Can you work these out from the drawing? Everything is in mm from the part's minimum corner. A direction names the side the tool comes from. Round coordinates to 2 decimals unless told otherwise and drop trailing zeros. Order: outer loops, then holes, each group sorted by start corner. A loop starts at its lowest first (then second) coordinate and runs counter-clockwise, first axis right, second up. Notation, with made-up numbers: (49.25, 75.5) -> (64.25, 75.5) arc R18 cw to (64.25, 92.5) -> close; hole circle Ø2 at (31, 22). An arc over 180 degrees is marked (long way). Use a Markdown table: item, result. Add a question column.
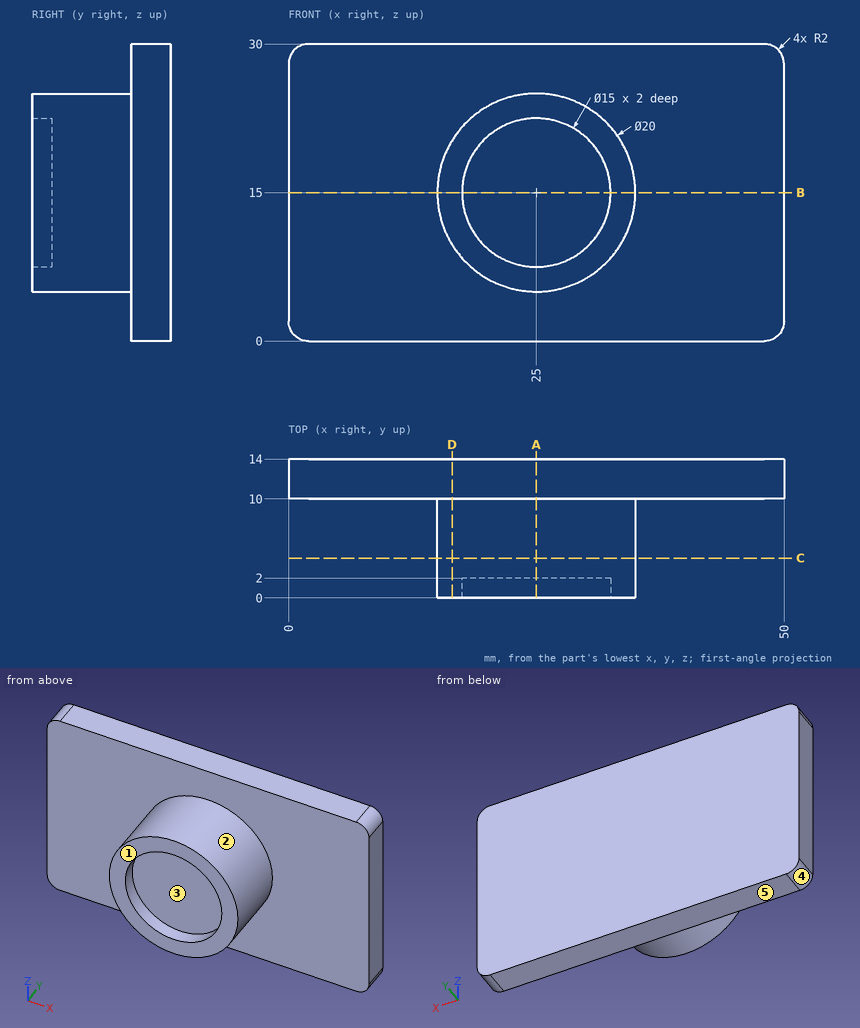
(1) I'm going to push flat-ended pins straight in: P1, Ø4, axis at x = 15.5, y = 2.5, coming from the -Z side; P2, Ø12, axis at x = 24, z = 15.5, coming from the -Y side; P3, Ø8, axis at x = 6, z = 5, coming from the -Y side. Where does each tip first touch, or does it pass through?
(2) I want a section at B-B on z = 15. List the corners of the cut face in (x, y) for me.
(3) I want a section at C-C on y = 4. List the corners of the cut face in (x, z) for me, and give its area (3 significant figures).
(4) I want a section at D-D on x = 16.5. List the corners of the cut face in (y, z) for me, and give its area (3 significant figures).
(5) I want a section at A-A on x = 25. List the corners of the cut face in (y, z) for me, and give its area (3 significant figures).
(6) If we mould it in two halves opening along X, with no side actions, what happens to the marked faces 3, 4 and 5? For each: pulls with the +X half, pulls with the -X half, needs draft (parallel to the pull), parting line crosses it, or undercut.
(7) On a 3-axis mill with a long thin cutter (end or side, diameter ignored), from which of +Z, -Z, +X, -X, +Y, -Y can I reach the whole of each face in a straight line? I mean the marked faces 1 and 2. Say none if no direction works.
(8) Please list where these lines run through material, in increasing order: probe 1 along Z at (x, y) = (25, 1.45); probe 2 along Y at (x, z) = (4, 10.5); probe 3 along Y at (x, z) = (27, 14.75). Write a range as from..to.
Output:
| question | item | result |
|---|---|---|
| 1 | P1 | z = 8.39 |
| 1 | P2 | y = 2 |
| 1 | P3 | y = 10 |
| 2 | outline | (0, 10) -> (15, 10) -> (15, 0) -> (17.5, 0) -> (17.5, 2) -> (32.5, 2) -> (32.5, 0) -> (35, 0) -> (35, 10) -> (50, 10) -> (50, 14) -> (0, 14) -> close |
| 3 | outline | circle Ø20 at (25, 15) |
| 3 | area | 314 mm² |
| 4 | outline | (0, 9.73) -> (10, 9.73) -> (10, 0) -> (14, 0) -> (14, 30) -> (10, 30) -> (10, 20.27) -> (0, 20.27) -> close |
| 4 | area | 225 mm² |
| 5 | outline | (0, 5) -> (10, 5) -> (10, 0) -> (14, 0) -> (14, 30) -> (10, 30) -> (10, 25) -> (0, 25) -> (0, 22.5) -> (2, 22.5) -> (2, 7.5) -> (0, 7.5) -> close |
| 5 | area | 290 mm² |
| 6 | face 3 | undercut |
| 6 | face 4 | pulls with the -X half |
| 6 | face 5 | needs draft |
| 7 | face 1 | +Z, -Z, +X, -X, -Y |
| 7 | face 2 | -Y |
| 8 | probe 1 | 5..7.5, 22.5..25 |
| 8 | probe 2 | 10..14 |
| 8 | probe 3 | 2..14 |
